Solid Edge part; units mm, degrees
sketch "Sketch1" plane through (0, 0, 0) normal (0, 0, 1) x (1, 0, 0)
  line L0 (57, -18) -> (57, 18)
  line L1 (57, 18) -> (-57, 18)
  line L2 (-57, 18) -> (-57, -18)
  line L3 (-57, -18) -> (57, -18)
extrude "Protrusion1" add sketch "Sketch1" along normal blind 5
sketch "Sketch2" plane through (-57, 0, 2.5) normal (-1, 0, 0) x (0, -1, 0)
  line L0 (-5, -0.5) -> (5, -0.5)
  line L1 (-8, 2.5) -> (8, 2.5)
  arc A0 (8, 2.5) -> (5, -0.5) centre (5, 2.5) cw
  arc A1 (-5, -0.5) -> (-8, 2.5) centre (-5, 2.5) cw
extrude "VaciadoExtruido_2" cut sketch "Sketch2" against normal blind 1
sketch "Sketch3" plane through (-56, 0, 2.5) normal (-1, 0, 0) x (0, -1, 0)
  line L0 (-5, -1.6) -> (5, -1.6)
  line L1 (-9.1, 2.5) -> (9.1, 2.5)
  arc A0 (9.1, 2.5) -> (5, -1.6) centre (5, 2.5) cw
  arc A1 (-5, -1.6) -> (-9.1, 2.5) centre (-5, 2.5) cw
extrude "VaciadoExtruido_3" cut sketch "Sketch3" against normal blind 112
fillet "Redondeo_3" radius 4.1 3 edges at (56, 7.8991, 2.1009) (56, -7.8991, 2.1009) (56, 0, 0.9)
sketch "Sketch4" plane through (0, 0, 5) normal (0, 0, 1) x (1, 0, 0)
  circle A0 centre (-53, 14) radius 1.6
extrude "Cutout1" cut sketch "Sketch4" against normal through all
sketch "Sketch5" plane through (0, 0, 0) normal (0, 0, -1) x (1, 0, 0)
  circle A0 centre (-53, -14) radius 3
extrude "VaciadoExtruido_5" cut sketch "Sketch5" against normal blind 3.5
pattern_linear "Pattern1" count 3 spacing 53 along (1, 0, 0) count 2 spacing 28 along (0, -1, 0) of "VaciadoExtruido_5", "Cutout1"
fillet "Redondeo_4" radius 4 4 edges at (-57, 18, 2.5) (-57, -18, 2.5) (57, 18, 2.5) (57, -18, 2.5)
Could you check a few things on this model? Use its own coordinates, in mm. A direction names the side the tool comes from. Give positions to 0.01 mm unless a question says otherwise; leave off trailing zeros. Loops run counter-clockwise (first coordinate to the right, second up) from the corner with the lowest first, then second, coordinate; pieces in that order, holes last. Notation, with made-up numbers: (68, 81.25) -> (123, 81.25) arc R28 ccw to (123, 103.25) -> close; hole circle Ø8 at (-37, -26.75). An arc over 180 degrees is marked (long way). Answer as CSV lines item,"result". Start each with the question number.
(1) If we section it at C-C on x = 33: Write out the boundary of the cut face in (y, z), then the cut area to 3 significant figures.
(2) I'm going to push flat-ended pins straight in: pin 1 Ø5 at (x, y) = (0, -14) entering from -Z; pin 2 Ø2.5 at (x, y) = (53, 14) entering from +Z; pin 3 Ø4 at (x, y) = (-44.5, -2) entering from +Z; pin 4 Ø8 at (x, y) = (15, 2.5) entering from +Z. Where does each tip first touch, or does it pass through?
(3) We'd pull the mould along X, two halves only. Please class faces 6 (the cylindrical face through (-0.65, -11.07, 1.73)), 7 (the cylindrical face through (-55.797, 16.859, 2.535)), 8 (the flat face through (1, 18, 2)): released by +X, released by -X, zero draft, split by the parting line, or undercut.
(4) If we section it at A-A on x = 0: Write out the boundary of the cut face in (y, z).
(5) Which directions (+Z, -Z, +X, -X, +Y, -Y) give clear straight access to the entire face, cutting with the end or side of a thin tool? Please do faces 1 (the cylindrical face through (54.526, 14.481, 4.26)), 2 (the flat face through (57, 0, 2)), 3 (the cylindrical face through (-56, -14, 2)), 4 (the cylindrical face through (-56.51, -7.1, 2.86)), 5 (the cylindrical face through (54.8, 0.1, 2.1)).
(6) I need wall thicknesses on probe 1 along X at (y, z) = (-14, 1.2); probe 2 along Y at (x, z) = (14, 4.7); probe 3 along Y at (x, z) = (-53, 4.15). Which ranges of each line are inside material? Lowest first, please.
Computed:
1,outline,"(-18, 0) -> (18, 0) -> (18, 5) -> (9.1, 5) arc R4.1 cw to (5, 0.9) -> (-5, 0.9) arc R4.1 cw to (-9.1, 5) -> (-18, 5) -> close"
1,area,"113 mm2"
2,pin 1,"stops at z = 3.5"
2,pin 2,"passes through"
2,pin 3,"stops at z = 0.9"
2,pin 4,"stops at z = 1.18"
3,face 6,"undercut"
3,face 7,"released by -X"
3,face 8,"zero draft"
4,outline,"(-18, 0) -> (-17, 0) -> (-17, 3.5) -> (-15.6, 3.5) -> (-15.6, 5) -> (-18, 5) -> close; (-12.4, 3.5) -> (-11, 3.5) -> (-11, 0) -> (11, 0) -> (11, 3.5) -> (12.4, 3.5) -> (12.4, 5) -> (9.1, 5) arc R4.1 cw to (5, 0.9) -> (-5, 0.9) arc R4.1 cw to (-9.1, 5) -> (-12.4, 5) -> close; (15.6, 3.5) -> (17, 3.5) -> (17, 0) -> (18, 0) -> (18, 5) -> (15.6, 5) -> close"
5,face 1,"+Z, -Z"
5,face 2,"+Z, -Z, +X, +Y, -Y"
5,face 3,"-Z"
5,face 4,"+Z, -X"
5,face 5,"+Z"
6,probe 1,"x = -57 to -56, -50 to -3, 3 to 50, 56 to 57"
6,probe 2,"y = -18 to -9.09, 9.09 to 18"
6,probe 3,"y = -18 to -15.6, -12.4 to -9.01, 9.01 to 12.4, 15.6 to 18"
